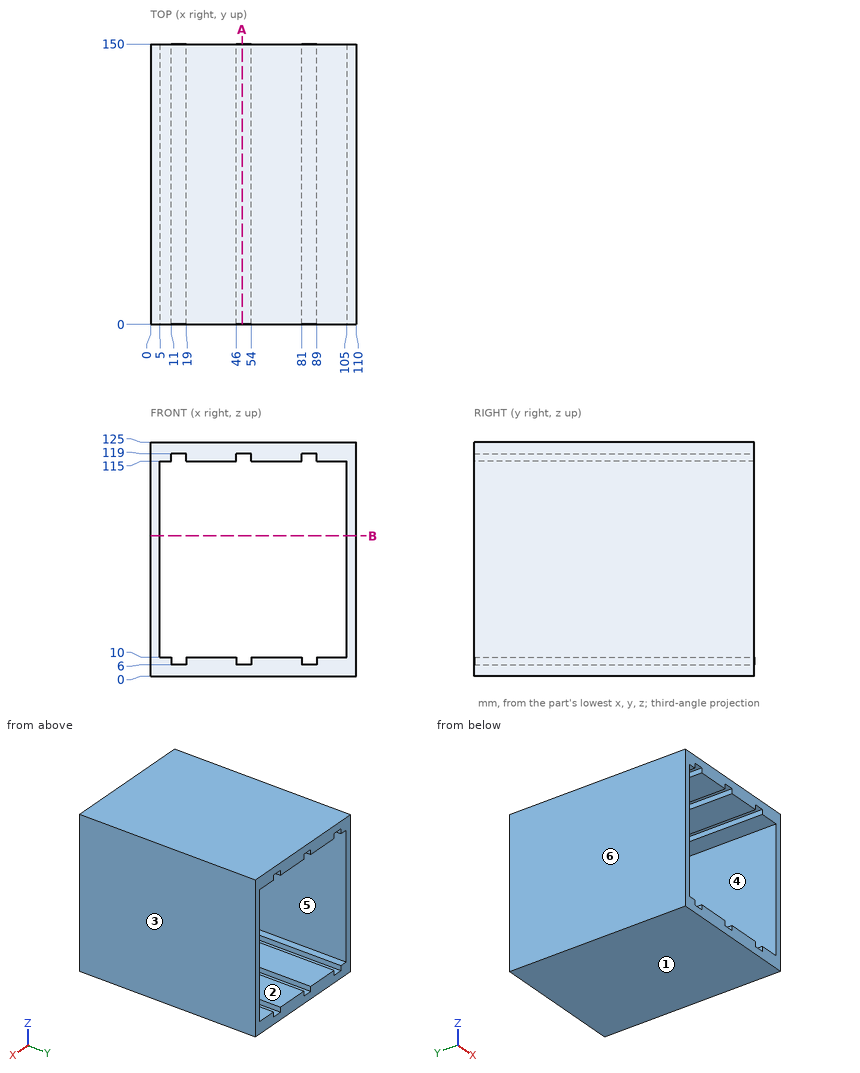
Could you check a few things on this drawing? It's one solid part, dimensions in mm from its lowest x, y, z. A direction names the side the tool comes from. Round coordinates to 2 decimals unless told otherwise and drop trailing zeros. Loops run counter-clockwise (first coordinate to the right, second up) from the corner with the lowest first, then second, coordinate; pieces in that order, holes last.
Q1. Thinking about a two-plate mould opening in X: for the marked faces 3, 4, 5 and 6, which applies, pulls with the +X half, pulls with the -X half, needs draft (parallel to the pull), parting line crosses it, or undercut?
Q2. On a 3-axis mill with a long thin cutter (end or side, diameter ignored), from which of +Z, -Z, +X, -X, +Y, -Y can I reach the whole of each face in a straight line? I mean the marked faces 1 and 2. Say none if no direction works.
Q3. I want a section at B-B (z = 75). Write out the boundary of the cut face in (x, y), and give its area (3 significant figures).
Q4. Please list where these lines run through material, in increasing order: L1, parallel to X at y = 32, z = 91.5; L2, parallel to Z at x = 96, y = 40; L3, parallel to Z at x = 84, y = 11.5.
Q5. I want a section at A-A (x = 49). Write out the boundary of the cut face in (y, z), and give its area (3 significant figures).
Answer below:
1. face 3: pulls with the +X half
1. face 4: undercut
1. face 5: undercut
1. face 6: pulls with the -X half
2. face 1: -Z, +X, -X, +Y, -Y
2. face 2: +Y, -Y
3. outline: (0, 0) - (5, 0) - (5, 150) - (0, 150) - close; (105, 0) - (110, 0) - (110, 150) - (105, 150) - close
3. area: 1,500 mm2
4. L1: x = 0 to 5, 105 to 110
4. L2: z = 0 to 10, 115 to 125
4. L3: z = 0 to 6, 119 to 125
5. outline: (0, 0) - (150, 0) - (150, 6) - (0, 6) - close; (0, 119) - (150, 119) - (150, 125) - (0, 125) - close
5. area: 1,800 mm2
